Autodesk Inventor part; units mm, degrees
ref_plane "YZ Plane" through (0, 0, 0) normal (1, 0, 0) x (0, 1, 0)
ref_plane "XZ Plane" through (0, 0, 0) normal (0, 1, 0) x (-1, 0, 0)
ref_plane "XY Plane" through (0, 0, 0) normal (0, 0, 1) x (1, 0, 0)
sketch "Skizze1" plane through (0, 0, 0) normal (0, 1, 0) x (-1, 0, 0)
  circle A0 centre (0, 0) radius 14
  circle A1 centre (0, 0) radius 17.5
  dimension "d0" = 28
  dimension "d1" = 35
extrude "Extrusion1" add sketch "Skizze1" along normal blind 100
sketch "Skizze2" plane through (0, 100, 0) normal (0, 1, 0) x (1, 0, 0)
  circle A0 centre (0, 0) radius 17.5 construction
  line L0 (-17.5, 0) -> (17.5, 0) construction
  line L1 (0, -17.5) -> (0, 17.5) construction
  line L2 (11.1238, 0) -> (19.1238, 0)
  line L3 (19.1238, 0) -> (19.1238, 0.5)
  line L4 (19.1238, 0.5) -> (11.1238, 0.5)
  line L5 (11.1238, 0.5) -> (11.1238, 0)
  line L6 (11.1238, 0) -> (19.1238, 0)
  line L7 (19.1238, 0) -> (19.1238, -0.5)
  line L8 (19.1238, -0.5) -> (11.1238, -0.5)
  line L9 (11.1238, -0.5) -> (11.1238, 0)
  dimension "d4" = 8
  dimension "d5" = 0.5
  dimension "d6" = 0.5
extrude "Extrusion2" cut sketch "Skizze2" against normal blind 1000
sketch "Skizze3" plane through (0, 100, 0) normal (0, 1, 0) x (1, 0, 0)
  arc A0 (17.4929, 0.5) -> (17.4929, -0.5) centre (0, 0) ccw construction
  line L0 (-17.5, 0) -> (17.4929, 0) construction
  line L1 (-17.5, 0) -> (-16.5, 0)
  line L2 (-16.5, 0) -> (-16.5, 10)
  line L3 (-16.5, 10) -> (-17.5, 10)
  line L4 (-17.5, 10) -> (-17.5, 0)
  line L5 (-17.5, 0) -> (-16.5, 0)
  line L6 (-16.5, 0) -> (-16.5, -14.1837)
  line L7 (-16.5, -14.1837) -> (-17.5, -14.1837)
  line L8 (-17.5, -14.1837) -> (-17.5, 0)
  line L9 (-0.0036, -17.5) -> (-0.0036, 17.5) construction
  line L10 (17.4929, 0) -> (16.4929, 0)
  line L11 (16.4929, 0) -> (16.4929, 10)
  line L12 (16.4929, 10) -> (17.4929, 10)
  line L13 (17.4929, 10) -> (17.4929, 0)
  line L14 (17.4929, 0) -> (16.4929, 0)
  line L15 (16.4929, 0) -> (16.4929, -14.1837)
  line L16 (16.4929, -14.1837) -> (17.4929, -14.1837)
  line L17 (17.4929, -14.1837) -> (17.4929, 0)
  dimension "d9" = 1
  dimension "d10" = 10
extrude "Extrusion3" cut sketch "Skizze3" against normal blind 1000
sketch "Skizze4" plane through (16.4929, 100, 5.8511) normal (1, 0, 0) x (0, 0, -1)
  line L0 (0, -100) -> (0, 0)
  line L1 (5.3511, 0) -> (0, 0)
  line L2 (0, 0) -> (0, -5)
  line L3 (0, -5) -> (5.3511, -5)
  line L4 (5.3511, -5) -> (5.3511, 0)
  line L5 (0, -5) -> (5.3511, -5)
  line L6 (5.3511, -5) -> (5.3511, -20)
  line L7 (5.3511, -20) -> (0, -20)
  line L8 (0, -20) -> (0, -5)
  line L9 (11.7023, 0) -> (11.7023, -100)
  line L10 (6.3511, 0) -> (11.7023, 0)
  line L11 (11.7023, 0) -> (11.7023, -5)
  line L12 (11.7023, -5) -> (6.3511, -5)
  line L13 (6.3511, -5) -> (6.3511, 0)
  line L14 (6.3511, -5) -> (11.7023, -5)
  line L15 (11.7023, -5) -> (11.7023, -20)
  line L16 (11.7023, -20) -> (6.3511, -20)
  line L17 (6.3511, -20) -> (6.3511, -5)
  line L18 (0, -50) -> (11.7023, -50) construction
  line L19 (5.3511, -100) -> (0, -100)
  line L20 (0, -100) -> (0, -95)
  line L21 (0, -95) -> (5.3511, -95)
  line L22 (5.3511, -95) -> (5.3511, -100)
  line L23 (0, -95) -> (5.3511, -95)
  line L24 (5.3511, -95) -> (5.3511, -80)
  line L25 (5.3511, -80) -> (0, -80)
  line L26 (0, -80) -> (0, -95)
  line L27 (6.3511, -100) -> (11.7023, -100)
  line L28 (11.7023, -100) -> (11.7023, -95)
  line L29 (11.7023, -95) -> (6.3511, -95)
  line L30 (6.3511, -95) -> (6.3511, -100)
  line L31 (6.3511, -95) -> (11.7023, -95)
  line L32 (11.7023, -95) -> (11.7023, -80)
  line L33 (11.7023, -80) -> (6.3511, -80)
  line L34 (6.3511, -80) -> (6.3511, -95)
  point P0 (5.8511, -100)
  point P1 (11.7023, -80)
  point P2 (0, -80)
  dimension "d13" = 5
  dimension "d14" = 15
  dimension "d15" = 15
extrude "Extrusion4" add sketch "Skizze4" along normal blind 15 contours L0 L3 L6 L7 | L0 L25 L24 L21 | L9 L29 L34 L33 | L9 L16 L17 L12
fillet "Rundung1" radius 2.5 8 edges at (31.4929, 95, 3.1756) (31.4929, 80, 3.1756) (31.4929, 80, -3.1756) (31.4929, 95, -3.1756) (31.4929, 20, 3.1756) (31.4929, 5, 3.1756) (31.4929, 20, -3.1756) (31.4929, 5, -3.1756)
sketch "Skizze5" plane through (16.4929, 80, 5.8511) normal (0, 0, 1) x (1, 0, 0)
  line L0 (0, 0) -> (12.5, 0) construction
  line L1 (0, 0) -> (7.5, 0) construction
  line L2 (0, 0) -> (7.5, 0) construction
  line L3 (7.5, 0) -> (7.5, 7.5) construction
  circle A0 centre (7.5, 7.5) radius 5
  line L4 (0, -75) -> (12.5, -75) construction
  line L5 (0, -75) -> (7.5, -75) construction
  line L6 (0, -75) -> (7.5, -75) construction
  line L7 (7.5, -75) -> (7.5, -67.5) construction
  circle A1 centre (7.5, -67.5) radius 5
  point P0 (-16.4929, -80)
  dimension "d19" = 7.5
  dimension "d20" = 0
  dimension "d21" = 7.5
  dimension "d22" = 90
  dimension "d23" = 10
  dimension "d24" = 7.5
  dimension "d25" = 0
  dimension "d26" = 7.5
  dimension "d27" = 90
  dimension "d28" = 10
extrude "Extrusion5" cut sketch "Skizze5" against normal blind 100
properties part number "Hülse"
Work out the finished part from the listing and answer in its coordinate system (mm). A direction names the side the tool comes from. Give positions to 0.01 mm unless a question says otherwise; leave off trailing zeros. Order: outer loops, then holes, each group sorted by start corner. A loop starts at its lowest first (then second) coordinate and runs counter-clockwise, first axis right, second up. Notation, with made-up numbers: (77, 66) -> (107, 66) arc R13 ccw to (107, 91) -> close; hole circle Ø11 at (73.25, -33.75). An arc over 180 degrees is marked (long way). Answer as a JSON object with one key per item and string values. Group by question number.
1. Consider line 1 along Z through (x, y) = (19.5, 91); line 2 along X through (y, z) = (86.5, -3); line 3 along Z through (x, y) = (3.5, 40). Determine where each line is inside the solid, lowest interval first. Write a range as [from, to].
2. Flat-ended cylindrical pins translate along their axes: pin 1 Ø6 at (x, y) = (23.99, 87.5) entering from +Z; pin 2 Ø4.5 at (x, z) = (24, -2) entering from -Y; pin 3 Ø5.5 at (y, z) = (2, -4) entering from +X; pin 4 Ø10 at (x, y) = (19.5, 25.5) entering from -Z. Find the tip coordinate at first contact, or state that the pin passes through.
3. Section A-A on y = 12.5 is taken. Count the separate pieces of the cut face and the enclosed holes in it, plus the area to 3 significant figures.
4. A tool of negligible diameter and unlimited length cuts with its end or side. For faces 1 (the flat face through (16.493, 3, 3)), 2 (the flat face through (16, 50, -0.5)), 3 (the cylindrical face through (30.78, 19.25, -3.14)), from which of +Z, -Z, +X, -X, +Y, -Y can it reach the whole face along a straight path? Write none if from no direction.
5. Section B-B on x = 0 is taken. Determine the outline of the cut face in (y, z).
6. Section C-C on z = 7 is taken. Determine the outline of the cut face in (x, y).
7. The mould has two halves that part along X. Classify faces 4 (the flat face through (24, 82, 5.851)), 5 (the flat face through (16.493, 50, 3)), 6 (the cylindrical face through (22.91, 82.62, -3.14)): released by +X, released by -X, zero draft, split by the parting line, or undercut.
Result sheet:
{
 "1": {"line 1": "z = [-5.85, -0.5], [0.5, 5.85]", "line 2": "x = [-16.5, -13.67], [13.67, 19.09], [28.89, 31.49]", "line 3": "z = [-17.15, -13.56], [13.56, 17.15]"},
 "2": {"pin 1": "passes through", "pin 2": "stops at y = 5", "pin 3": "stops at x = 16.49", "pin 4": "stops at z = -9.8"},
 "3": {"separate pieces": "3", "enclosed holes": "0", "area": "382 mm^2"},
 "4": {"face 1": "+Z, -Z, +X, -Y", "face 2": "+X, +Y, -Y", "face 3": "+Z, -Z, +X"},
 "5": {"outline": "(0, -17.5) -> (100, -17.5) -> (100, -14) -> (0, -14) -> close; (0, 14) -> (100, 14) -> (100, 17.5) -> (0, 17.5) -> close"},
 "6": {"outline": "(-16.04, 0) -> (-12.12, 0) -> (-12.12, 100) -> (-16.04, 100) -> close; (12.12, 0) -> (16.04, 0) -> (16.04, 100) -> (12.12, 100) -> close"},
 "7": {"face 4": "zero draft", "face 5": "released by +X", "face 6": "undercut"}
}
